Input: part model. Units: mm. Frame: model coordinates. Face numbers are marked on the shaded views. A direction names the side the tool comes from. Round coordinates to 2 decimals unless told otherwise and drop trailing zeros. Loops run counter-clockwise (first coordinate to the right, second up) from the corner with the lowest first, then second, coordinate; pieces in that order, holes last. Notation, with made-up numbers: (69.25, -17.75) - (117.25, -17.75) arc R12 ccw to (117.25, -3.75) - close; hole circle Ø8 at (-9, 13). An arc over 180 degrees is marked (long way). Use CSV: the item, a comma, the result in double quotes. Start each with the question number.
1. Pull-direction query (X, two-part tool) for the marked faces 3 and 4; classes: +X half, -X half, draft (parallel to the pull), parting line (faces both ways), or undercut.
2. Cut plane A-A (x = 0). Return loops of the section in (y, z).
3. Material intervals for probe 1 along X at (y, z) = (2.2, 0); probe 2 along X at (y, z) = (1.5, -24); probe 3 along Y at (x, z) = (-16, -12.5), sorted ascending. Write a range as from..to.
4. Cut plane B-B (y = 6.75). Return loops of the section in (x, z) (3 decimals), and give its area (3 significant figures).
5. Pin query (flat end, axial travel): P1, Ø2, axis at x = -19, z = 24.5, coming from the -Y side; P2, Ø2, axis at x = -9, y = 7, coming from the +Z side; P3, Ø4, axis at y = 4, z = 26.5, coming from the +X side; P4, Ø2.5, axis at x = 4, y = 3, coming from the +Z side. Return the tip coordinate at first contact, or that it passes through.
6. Cut plane C-C (z = 0). Return loops of the section in (x, y).
7. Access query for the marked faces 1 and 2. Directions: +Z, -Z, +X, -X, +Y, -Y. A direction counts if a zero-diameter tool reaches every point of the face in a straight line with its end or side. Return the directions, or none.
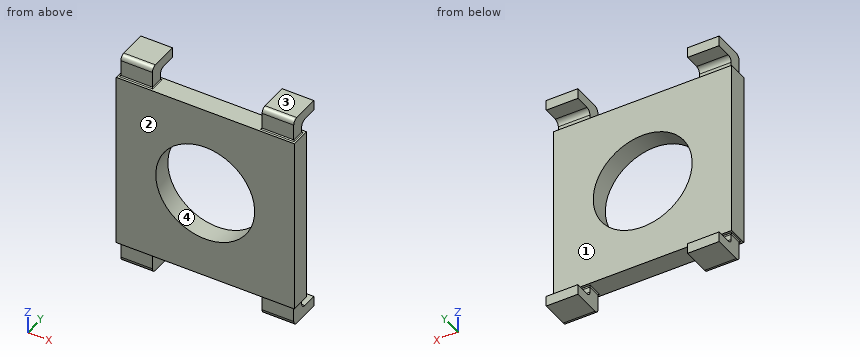
```python
from build123d import *

# Parameters (mm, degrees)
SKETCH2_W           = 45
SKETCH2_H           = 45
BOSS_EXTRUDE1_DEPTH = 5
SKETCH3_W           = 8
SKETCH3_H           = 3.3
BOSS_EXTRUDE2_DEPTH = 28
FILLET1_R           = 0.25
SKETCH4_W           = 8
SKETCH4_H           = 2.625
BOSS_EXTRUDE3_DEPTH = 5
FILLET2_R           = 1.25
SKETCH6_R           = 12.5
CUT_EXTRUDE1_DEPTH  = 19


with BuildPart() as part:
    # Sketch2 → Boss-Extrude1 (new body)
    with BuildSketch(Plane(origin=(0, 0, 0), x_dir=(1, 0, 0), z_dir=(0, 1, 0))):
        Rectangle(SKETCH2_W, SKETCH2_H)
    extrude(amount=BOSS_EXTRUDE1_DEPTH)

    # Sketch3 → Boss-Extrude2 (add, symmetric)
    with BuildSketch(Plane.XY):
        with Locations((-17.853613933, 2.5)):
            Rectangle(SKETCH3_W, SKETCH3_H)
        with Locations((17.853613933, 2.5)):
            Rectangle(SKETCH3_W, SKETCH3_H)
    extrude(amount=BOSS_EXTRUDE2_DEPTH, both=True)

    # Fillet1
    fillet1_edges = [part.edges().sort_by_distance(p)[0] for p in [
        (21.853613933, 2.5, 22.5),
        (17.853613933, 0.85, 22.5),
        (13.853613933, 2.5, 22.5),
        (17.853613933, 4.15, 22.5),
        (-17.853613933, 0.85, 22.5),
        (-21.853613933, 2.5, 22.5),
        (-17.853613933, 4.15, 22.5),
        (-13.853613933, 2.5, 22.5),
        (-13.853613933, 2.5, -22.5),
        (-17.853613933, 4.15, -22.5),
        (-21.853613933, 2.5, -22.5),
        (-17.853613933, 0.85, -22.5),
        (17.853613933, 4.15, -22.5),
        (13.853613933, 2.5, -22.5),
        (17.853613933, 0.85, -22.5),
        (21.853613933, 2.5, -22.5),
    ]]
    fillet(fillet1_edges, radius=FILLET1_R)

    # Sketch4 → Boss-Extrude3 (add)
    with BuildSketch(Plane(origin=(0, 4.15, 0), x_dir=(1, 0, 0), z_dir=(0, 1, 0))):
        with Locations((-17.853613933, 26.6875)):
            Rectangle(SKETCH4_W, SKETCH4_H)
        with Locations((17.853613933, 26.6875)):
            Rectangle(SKETCH4_W, SKETCH4_H)
        with Locations((17.853613933, -26.6875)):
            Rectangle(SKETCH4_W, SKETCH4_H)
        with Locations((-17.853613933, -26.6875)):
            Rectangle(SKETCH4_W, SKETCH4_H)
    extrude(amount=BOSS_EXTRUDE3_DEPTH)

    # Fillet2
    fillet2_edges = [part.edges().sort_by_distance(p)[0] for p in [
        (-17.853613933, 4.15, 25.375),
        (17.853613933, 4.15, 25.375),
        (17.853613933, 4.15, -25.375),
        (-17.853613933, 4.15, -25.375),
        (-17.853613933, 0.85, -28),
        (-17.853613933, 0.85, 28),
        (17.853613933, 0.85, -28),
        (17.853613933, 0.85, 28),
    ]]
    fillet(fillet2_edges, radius=FILLET2_R)

    # Sketch6 → Cut-Extrude1 (cut)
    with BuildSketch(Plane(origin=(0, 5, 0), x_dir=(1, 0, 0), z_dir=(0, 1, 0))):
        with Locations(Location((0, 0, 0), (0, 0, 270))):
            Circle(SKETCH6_R)
    extrude(amount=-CUT_EXTRUDE1_DEPTH, mode=Mode.SUBTRACT)


solid = part.part
```
Established:
1,face 3,"draft"
1,face 4,"undercut"
2,outline,"(0, -22.5) - (5, -22.5) - (5, -12.5) - (0, -12.5) - close; (0, 12.5) - (5, 12.5) - (5, 22.5) - (0, 22.5) - close"
3,probe 1,"x = -22.5..-12.5, 12.5..22.5"
3,probe 2,"x = -21.85..-13.85, 13.85..21.85"
3,probe 3,"y = 0..5"
4,outline,"(-21.854, -28) - (-13.854, -28) - (-13.854, -25.375) - (-21.854, -25.375) - close; (-21.854, 25.375) - (-13.854, 25.375) - (-13.854, 28) - (-21.854, 28) - close; (13.854, -28) - (21.854, -28) - (21.854, -25.375) - (13.854, -25.375) - close; (13.854, 25.375) - (21.854, 25.375) - (21.854, 28) - (13.854, 28) - close"
4,area,"84.0 mm2"
5,P1,"stops at y = 0.85"
5,P2,"passes through"
5,P3,"stops at x = 21.85"
5,P4,"stops at z = 22.5"
6,outline,"(-22.5, 0) - (-12.5, 0) - (-12.5, 5) - (-22.5, 5) - close; (12.5, 0) - (22.5, 0) - (22.5, 5) - (12.5, 5) - close"
7,face 1,"+X, -X, +Y"
7,face 2,"+Z, -Z, +X, -X, -Y"
